For this review, take the finished solid that the model builds, in its own axes (mm). A direction names the side the tool comes from. Coordinates: 2 decimals unless noted, no trailing zeros. Loops run counter-clockwise (first coordinate to the right, second up) from the corner with the lowest first, then second, coordinate; pieces in that order, holes last. Notation, with made-up numbers: M 68,-6.75 L 124,-6.75 A14 cw 124,19.25 Z; hole C -20,-4 d8. An arc over 180 degrees is marked long. Answer as a JSON object with one key per item and string values. Group by question number.
Item 1: Add section A-A (x = -60). State the section outline as (y, z) points.
Item 2: Add section B-B (z = -10). State the section outline as (x, y) points.
Item 3: Insertion check: pin 1 (3 mm diameter, centred on x = 54.5, y = -24.5, fed in from +Z); pin 2 (5 mm diameter, centred on x = -34, y = 67.5, fed in from -Z); pin 3 (22 mm diameter, centred on x = -47, z = -14.5, fed in from -Y). Each pin has a flat end and moves straight along its axis. Give the tip position at first contact, or say it passes through.
Item 4: Mouldability with a two-part tool opening along Z and no side actions: class faces 4 (the face through (138.54, 70.07, -40.07)), 5 (the face through (94.7, 15.6, -8)), 6 (the face through (-75, 18, 1)) as +Z half, -Z half, draft (parallel to the pull), parting line (faces both ways), or undercut.
Item 5: Wall thickness on L1, parallel to Y at x = -57.5, z = -18; L2, parallel to Z at x = 21, y = -61; L3, parallel to Z at x = 27, y = -1: over which ranges is each line inside the solid? List them lowest first. Write a range as from..to.
Item 6: Add section C-C (y = -24.5). State the section outline as (x, z) points, then the cut area to 3 significant figures.
Item 7: Add section D-D (x = 81). State the section outline as (y, z) points.
Item 8: Tool access review of faces 1 (the face through (-20, 70, -10)), 2 (the face through (-47, 65, -10)), 3 (the face through (-47, 70, -20)): name each direction out of +Z, -Z, +X, -X, +Y, -Y from which nothing blocks a thin tool from reaching the whole face with its end or side.
from build123d import *

# Parameters (mm, degrees)
SKETCH_1_W          = 50
SKETCH_1_H          = 150
EXTRUDE_1_DEPTH     = 10
SKETCH_3_W          = 10
SKETCH_3_H          = 150
EXTRUDE_2_DEPTH     = 280
EXTRUDE_3_DEPTH     = 10
CUT_EXTRUDE_1_DEPTH = 50
EXTRUDE_4_DEPTH     = 50
SKETCH_9_R          = 4
CUT_EXTRUDE_2_DEPTH = 30
CUT_EXTRUDE_4_DEPTH = 10


with BuildPart() as part:
    # Sketch 1 → Extrude 1 (new body)
    with BuildSketch(Plane.XY):
        Rectangle(SKETCH_1_W, SKETCH_1_H)
    extrude(amount=EXTRUDE_1_DEPTH)



with BuildPart() as body_2:
    # Sketch 3 → Extrude 2 (new body)
    with BuildSketch(Plane(origin=(25, 75, 0), x_dir=(-0.2544932992796438, 0, -0.9670745372626465), z_dir=(0.9670745372626465, 0, -0.2544932992796438))):
        with Locations((-5, -75)):
            Rectangle(SKETCH_3_W, SKETCH_3_H)
    extrude(amount=EXTRUDE_2_DEPTH)


with BuildPart() as part_1:
    add(part.part)

    add(body_2.part)  # Loft 8 merges body 2
    # Sketch 4 → Loft 8 section 0
    with BuildSketch(Plane(origin=(25, 0, 0), x_dir=(0, 0, -1), z_dir=(1, 0, 0))):
        with BuildLine():
            Line((-10, 75), (0, 75))
            Line((0, 75), (0, -75))
            Line((0, -75), (-10, -75))
            Line((-10, -75), (-10, 75))
        make_face()
    # Sketch 5 → Loft 8 section 1
    with BuildSketch(Plane(origin=(23.380829016, 0, -6.152849741), x_dir=(0.25449329927964376, 0, 0.9670745372626466), z_dir=(-0.9670745372626466, 0, 0.25449329927964376))):
        with BuildLine():
            Line((6.362332482, 75), (16.362332482, 75))
            Line((16.362332482, 75), (16.362332482, -75))
            Line((16.362332482, -75), (6.362332482, -75))
            Line((6.362332482, -75), (6.362332482, 75))
        make_face()
    loft()

    # Sketch 6 → Extrude 3 (add)
    with BuildSketch(Plane(origin=(0, 75, 0), x_dir=(1, 0, 0), z_dir=(0, 1, 0))):
        Polygon((25, 0), (295.780870434, 71.258123798), (290.691004448, 90.599614544), (22.412469182, 20), (-25, 20), (-25, 0), align=None)
    extrude(amount=-EXTRUDE_3_DEPTH)

    # Sketch 7 → Cut-Extrude 1 (cut, symmetric)
    with BuildSketch(Plane(origin=(1.619170984, 0, 6.152849741), x_dir=(-0.9670745372626465, 0, 0.2544932992796438), z_dir=(-0.2544932992796438, 0, -0.9670745372626465))):
        Polygon((-194.176863432, 65), (-24.176863432, -77.6469373), (26.721796424, -75), (44.26157498, -115.472113567), (-316.323525899, -105.286880986), (-321.035103343, 79.29609417), (-302.302762067, 102.681692196), (-235.315396996, 89.416867429), (-227.148078723, 92.666134591), align=None)
    extrude(amount=CUT_EXTRUDE_1_DEPTH, both=True, mode=Mode.SUBTRACT)

    # Sketch 8 → Extrude 4 (add)
    with BuildSketch(Plane.ZY.offset(25)):
        Polygon((0, 65), (0, -75), (10, -75), (10, 75), (-20, 75), (-20, 65), align=None)
    extrude(amount=EXTRUDE_4_DEPTH)

    # Sketch 9 → Cut-Extrude 2 (cut)
    with BuildSketch(Plane.XZ.offset(-65)):
        with Locations(Location((-60, -10, 0), (0, 0, 270))):
            Circle(SKETCH_9_R)
        with Locations(Location((-30, -10, 0), (0, 0, 270))):
            Circle(SKETCH_9_R)
        with Locations(Location((178.459459466, -45.554300571, 0), (0, 0, 270))):
            Circle(SKETCH_9_R)
        with Locations(Location((149.447223348, -37.919501593, 0), (0, 0, 270))):
            Circle(SKETCH_9_R)
    extrude(amount=-CUT_EXTRUDE_2_DEPTH, mode=Mode.SUBTRACT)

    # Sketch 10 → Cut-Extrude 4 (cut)
    with BuildSketch(Plane(origin=(0, 75, 0), x_dir=(1, 0, 0), z_dir=(0, 1, 0))):
        Polygon((141.048944472, 30.539195914), (135.959078486, 49.880686659), (22.412469182, 20), (-20, 20), (-20, 0), (25, 0), align=None)
    extrude(amount=-CUT_EXTRUDE_4_DEPTH, mode=Mode.SUBTRACT)


solid = part_1.part
From the geometry:
{
 "1": {"outline": "M -75,0 L 65,0 L 65,-6 L 75,-6 L 75,10 L -75,10 Z; M 65,-20 L 75,-20 L 75,-14 L 65,-14 Z"},
 "2": {"outline": "M -75,65 L -64,65 L -64,75 L -75,75 Z; M -56,65 L -34,65 L -34,75 L -56,75 Z; M -26,65 L -20,65 L -20,75 L -26,75 Z; M 63,-44.68 L 102.29,-12.79 L 102.29,75 L 63,75 Z"},
 "3": {"pin 1": "stops at z = 2.97", "pin 2": "stops at z = -20", "pin 3": "stops at y = 65"},
 "4": {"face 4": "undercut", "face 5": "+Z half", "face 6": "draft"},
 "5": {"L1": "y = 65..75", "L2": "z = 0..10", "L3": "z = -0.53..9.74"},
 "6": {"outline": "M -75,0 L 25,0 L 86.25,-16.12 L 88.8,-6.45 L 27.54,9.67 L 25,10 L -75,10 Z", "area": "1,650 mm²"},
 "7": {"outline": "M -31.27,-4.4 L -29.06,-14.74 L 75,-14.74 L 75,-4.4 Z"},
 "8": {"face 1": "-Z, +Y, -Y", "face 2": "-Z, -X, -Y", "face 3": "-Z, -X, +Y, -Y"}
}
